Here's how the part is built. I have some questions about the finished solid (model axes, mm). Face numbers are marked on the shaded views. Round coordinates to 2 decimals unless told otherwise and drop trailing zeros. Write each loop counter-clockwise with the first axis right and the second up, starting at its lowest first coordinate (ties: lowest second). Pieces come first, ordered by that corner, then holes. Notation, with made-up numbers: (-25, 37) -> (20, 37) arc R27 cw to (20, 73) -> close; hole circle Ø11 at (6, 3). An arc over 180 degrees is marked (long way). Answer as CSV lines item,"result".
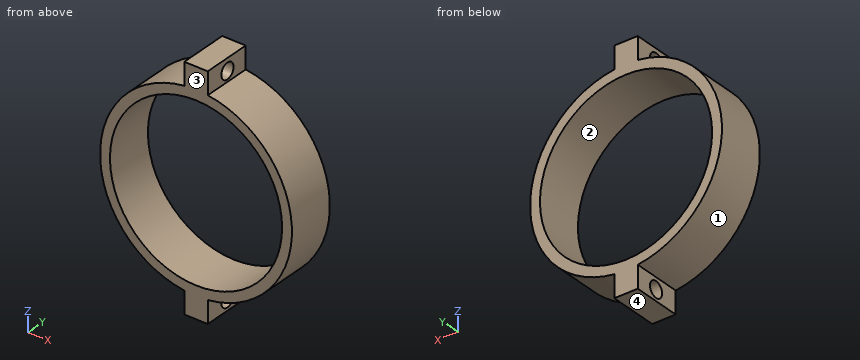
```python
from build123d import *

# Parameters (mm, degrees)
SKETCH2_R           = 19.5
SKETCH2_R_2         = 17.5
BOSS_EXTRUDE2_DEPTH = 10
SKETCH3_R           = 1.6
CUT_EXTRUDE1_DEPTH  = 10


with BuildPart() as part:
    # Sketch2 → Boss-Extrude2 (new body)
    # profile 1 of 3: a face of its own
    with BuildSketch(Plane(origin=(0, 0, 0), x_dir=(1, 0, 0), z_dir=(0, 1, 0))):
        Circle(SKETCH2_R)
        with Locations(Location((0, 0, 0), (0, 0, 270))):
            Circle(SKETCH2_R_2, mode=Mode.SUBTRACT)
    # profile 2 of 3: a face of its own
    with BuildSketch(Plane(origin=(0, 0, 0), x_dir=(1, 0, 0), z_dir=(0, 1, 0))):
        with BuildLine():
            ThreePointArc((-2.387522163, 19.353287522), (0, 19.5), (2.387522163, 19.353287522))
            Line((2.387522163, 19.353287522), (2.387522163, 23.886441242))
            Line((2.387522163, 23.886441242), (-2.387522163, 23.886441242))
            Line((-2.387522163, 23.886441242), (-2.387522163, 19.353287522))
        make_face()
    # profile 3 of 3: a face of its own
    with BuildSketch(Plane(origin=(0, 0, 0), x_dir=(1, 0, 0), z_dir=(0, 1, 0))):
        with BuildLine():
            Line((2.387522163, -23.886441242), (2.387522163, -19.353287522))
            ThreePointArc((2.387522163, -19.353287522), (0, -19.5), (-2.387522163, -19.353287522))
            Line((-2.387522163, -19.353287522), (-2.387522163, -23.886441242))
            Line((-2.387522163, -23.886441242), (2.387522163, -23.886441242))
        make_face()
    extrude(amount=BOSS_EXTRUDE2_DEPTH)

    # Sketch3 → Cut-Extrude1 (cut)
    with BuildSketch(Plane.ZY.offset(2.387522163)):
        with Locations((-21.687379423, 5.18275768)):
            Circle(SKETCH3_R)
        with Locations((21.434001351, 5.18275768)):
            Circle(SKETCH3_R)
    extrude(amount=-CUT_EXTRUDE1_DEPTH, mode=Mode.SUBTRACT)


solid = part.part
```
1. If I drill on line 1 (X direction, y = 2.75, z = 0); line 2 (X direction, y = 3.75, z = 14); line 3 (Z direction, x = -12, y = 8), over which ranges is the centre line in solid material (lowest first)?
Numbers:
line 1,"x = -19.5 to -17.5, 17.5 to 19.5"
line 2,"x = -13.57 to -10.5, 10.5 to 13.57"
line 3,"z = -15.37 to -12.74, 12.74 to 15.37"
2. For pin 1 Ø3.5 at (y, z) = (5.18, -21.69) entering from +X; pin 2 Ø3.5 at (y, z) = (3.5, -22.5) entering from -X; pin 3 Ø6 at (x, y) = (12.5, 6) entering from -Z; pin 4 Ø1.9 at (y, z) = (5.18, 21.43) entering from +X, each with a flat end and sliding along its axis, tell me the tip position at first contact or that it passes through.
Numbers:
pin 1,"stops at x = 2.39"
pin 2,"stops at x = -2.39"
pin 3,"stops at z = -17.03"
pin 4,"passes through"
3. Suppose I cut it at D-D on x = 0. Please give me the cut outline in (y, z).
Numbers:
outline,"(0, -23.89) -> (10, -23.89) -> (10, -17.5) -> (0, -17.5) -> close; (0, 17.5) -> (10, 17.5) -> (10, 23.89) -> (0, 23.89) -> close; hole circle Ø3.2 at (5.18, -21.69); hole circle Ø3.2 at (5.18, 21.43)"
4. Suppose I cut it at A-A on y = 8.75. Please give me the cut outline in (x, z).
Numbers:
outline,"(-2.39, -23.89) -> (2.39, -23.89) -> (2.39, -19.35) arc R19.5 ccw to (2.39, 19.35) -> (2.39, 23.89) -> (-2.39, 23.89) -> (-2.39, 19.35) arc R19.5 ccw to (-2.39, -19.35) -> close; hole circle Ø35 at (0, 0)"
5. Suppose I cut it at C-C on z = 10. Please give me the cut outline in (x, y).
Numbers:
outline,"(-16.74, 0) -> (-14.36, 0) -> (-14.36, 10) -> (-16.74, 10) -> close; (14.36, 0) -> (16.74, 0) -> (16.74, 10) -> (14.36, 10) -> close"
6. If we mould it in two halves opening along Z, with no side actions, what happens to the marked faces 1, 2, 3 and 4? For each: released by +Z, released by -Z, zero draft, split by the parting line, or undercut.
Numbers:
face 1,"split by the parting line"
face 2,"undercut"
face 3,"zero draft"
face 4,"released by -Z"
7. Suppose I cut it at B-B on x = -8. Please give me the cut outline in (y, z).
Numbers:
outline,"(0, -17.78) -> (10, -17.78) -> (10, -15.56) -> (0, -15.56) -> close; (0, 15.56) -> (10, 15.56) -> (10, 17.78) -> (0, 17.78) -> close"
